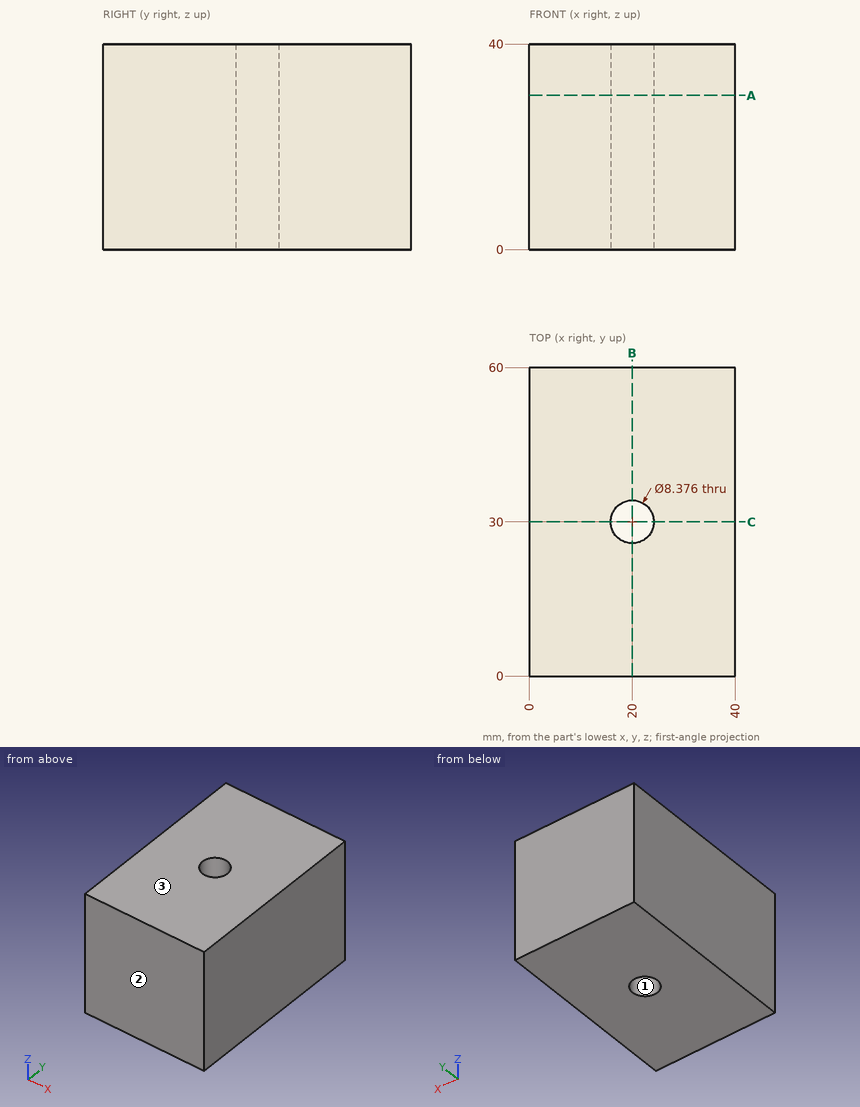
Study the drawing (mm; zero at the part's minimum x, y, z) and answer. Give positions to 0.01 mm unless a question says otherwise; leave off trailing zeros. Write each loop counter-clockwise with the first axis right and the second up, starting at its lowest first coordinate (ties: lowest second). Pieces come first, ordered by that corner, then holes. Notation, with made-up numbers: (-23.75, -20) - (27.25, -20) arc R33 cw to (27.25, 15) - close; hole circle Ø1 at (11.5, -4). An arc over 180 degrees is marked (long way). Use a Markdown table: item, result.
1. Section A-A on z = 30 is taken. Write down the section's boundary in (x, y), plus the area to 3 significant figures.
Values follow:
| item | result |
|---|---|
| outline | (0, 0) - (40, 0) - (40, 60) - (0, 60) - close; hole circle Ø8.38 at (20, 30) |
| area | 2,340 mm² |
2. For a pull along Y with two mould halves and no side action, classify the marked faces 1, 2 and 3 as released by +Y, released by -Y, zero draft, split by the parting line, or undercut.
Values follow:
| item | result |
|---|---|
| face 1 | undercut |
| face 2 | released by -Y |
| face 3 | zero draft |
3. Find the intervals of material crossed by probe 1 along X at (y, z) = (30, 12); probe 2 along Y at (x, z) = (20, 30); probe 3 along Y at (x, z) = (17.5, 14), in increasing order. Write a range as from..to.
Values follow:
| item | result |
|---|---|
| probe 1 | x = 0..15.81, 24.19..40 |
| probe 2 | y = 0..25.81, 34.19..60 |
| probe 3 | y = 0..26.64, 33.36..60 |
4. This flat-tipped pin is pushed along its axis until it touches: P1, Ø2, axis at y = 30, z = 34, coming from the -X side. Where does it stop, or does it pass through?
Values follow:
| item | result |
|---|---|
| P1 | stops at x = 0 |
5. Section C-C on y = 30 is taken. Write down the section's boundary in (x, z), plus the area to 3 significant figures.
Values follow:
| item | result |
|---|---|
| outline | (0, 0) - (15.81, 0) - (15.81, 40) - (0, 40) - close; (24.19, 0) - (40, 0) - (40, 40) - (24.19, 40) - close |
| area | 1,260 mm² |
6. Section B-B on x = 20 is taken. Write down the section's boundary in (y, z), plus the area to 3 significant figures.
Values follow:
| item | result |
|---|---|
| outline | (0, 0) - (25.81, 0) - (25.81, 40) - (0, 40) - close; (34.19, 0) - (60, 0) - (60, 40) - (34.19, 40) - close |
| area | 2,060 mm² |
